Source: CAD feature listing. Evaluate the final solid. Frame: model axes, mm. Round coordinates to 2 decimals unless told otherwise and drop trailing zeros. Order: outer loops, then holes, each group sorted by start corner. A loop starts at its lowest first (then second) coordinate and runs counter-clockwise, first axis right, second up. Notation, with made-up numbers: (46, 63) - (67, 63) arc R25 cw to (67, 92) - close; hole circle Ø2 at (-23.5, 46). An arc over 180 degrees is marked (long way). Return JSON: item names as keys, results as strings. Group by question number.
1) Contact query for a flat-ended pin moving along its axis: P1, Ø5, axis at x = 5, z = 54, coming from the +Y side. Output: stop coordinate, or through.
2) Section B-B, the plane z = -42. Return loops of the section in (x, y).
3) Section C-C, the plane y = -31. Return loops of the section in (x, z).
4) Ray query, line 1 (Y direction, x = 3.5, z = -32.5); line 2 (Z direction, x = 8, y = 30); line 3 (Y direction, x = 0.5, z = 1.5). Return the intervals inside material, ascending. Write a range as from..to.
5) Section A-A, the plane x = 6.5. Return loops of the section in (y, z).
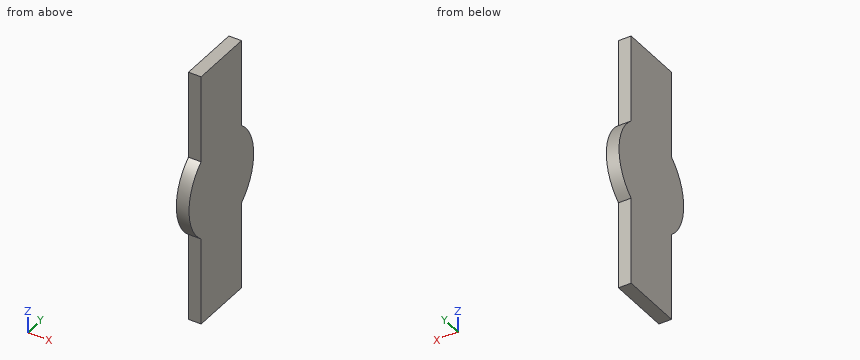
Autodesk Inventor part; units mm, degrees
ref_plane "YZ Plane" through (0, 0, 0) normal (1, 0, 0) x (0, 1, 0)
ref_plane "XZ Plane" through (0, 0, 0) normal (0, 1, 0) x (-1, 0, 0)
ref_plane "XY Plane" through (0, 0, 0) normal (0, 0, 1) x (1, 0, 0)
sketch "スケッチ1" plane through (0, 0, 0) normal (1, 0, 0) x (0, 1, 0)
  circle A0 centre (0, 0) radius 40
  line L0 (-25, 100) -> (25, 100)
  line L1 (25, 100) -> (25, -100)
  line L2 (25, -100) -> (-25, -100)
  line L3 (-25, -100) -> (-25, 100)
  line L4 (-25, 100) -> (25, -100) construction
  line L5 (25, 100) -> (-25, -100) construction
  point P0 (25, -31.225)
  point P1 (25, 31.225)
  point P2 (-25, 31.225)
  point P3 (-25, -31.225)
  dimension "d0" = 80
  dimension "d1" = 50
  dimension "d2" = 200
extrude "押し出し1" add sketch "スケッチ1" along normal blind 10
ref_plane "作業平面1" through (0, -25, 0) normal (0, 0, 1) x (1, 0, 0)
properties part number "leg_base_plate"
Geometry check:
{
 "1": {"P1": "y = 25"},
 "2": {"outline": "(0, -25) - (10, -25) - (10, 25) - (0, 25) - close"},
 "3": {"outline": "(0, -25.28) - (10, -25.28) - (10, 25.28) - (0, 25.28) - close"},
 "4": {"line 1": "-25..25", "line 2": "-26.46..26.46", "line 3": "-39.97..39.97"},
 "5": {"outline": "(-25, -100) - (25, -100) - (25, -31.22) arc R40 ccw to (25, 31.22) - (25, 100) - (-25, 100) - (-25, 31.22) arc R40 ccw to (-25, -31.22) - close"}
}
